```python
from build123d import *

# Parameters (mm, degrees)
SKETCH1_W                                    = 200
SKETCH1_H                                    = 40
BOSS_EXTRUDE1_DEPTH                          = 6
CSK_FOR_M6_COUNTERSUNK_FLAT_HEAD_SCR_2_COUNT = 2
CSK_FOR_M6_COUNTERSUNK_FLAT_HEAD_SCR_2_PITCH = 14
CSK_FOR_M6_COUNTERSUNK_FLAT_HEAD_SCR_3_COUNT = 2
CSK_FOR_M6_COUNTERSUNK_FLAT_HEAD_SCR_3_PITCH = 19.798989873
CSK_FOR_M6_COUNTERSUNK_FLAT_HEAD_SCR_4_COUNT = 2
CSK_FOR_M6_COUNTERSUNK_FLAT_HEAD_SCR_4_PITCH = 14
CHAMFER1_SIZE                                = 2
SKETCH8_R                                    = 5
CUT_EXTRUDE1_DEPTH                           = 103.156742313


with BuildPart() as part:
    # Sketch1 → Boss-Extrude1 (new body)
    with BuildSketch(Plane(origin=(0, 0, 0), x_dir=(1, 0, 0), z_dir=(0, 1, 0))):
        Rectangle(SKETCH1_W, SKETCH1_H)
    extrude(amount=BOSS_EXTRUDE1_DEPTH)

    # Sketch5 → CSK for M6 Countersunk Flat Head Screw1 (revolve, cut)
    with BuildSketch(Plane(origin=(-7, 6, -7), x_dir=(0, 0, 1), z_dir=(1, 0, 0))):
        Polygon((0, 0), (0, 6), (3.3, 6), (3.3, 3.2), (6.5, 0), align=None)
    csk_for_m6_countersunk_flat_head_screw1 = revolve(axis=Axis((-7, 12.35, -7), (0, -1, 0)), mode=Mode.SUBTRACT)

    # CSK for M6 Countersunk Flat Head Scr 2: CSK for M6 Countersunk Flat Head Screw1 ×2
    with Locations(*[(i * CSK_FOR_M6_COUNTERSUNK_FLAT_HEAD_SCR_2_PITCH, 0, 0) for i in range(1, CSK_FOR_M6_COUNTERSUNK_FLAT_HEAD_SCR_2_COUNT)]):
        add(csk_for_m6_countersunk_flat_head_screw1, mode=Mode.SUBTRACT)

    # CSK for M6 Countersunk Flat Head Scr 3: CSK for M6 Countersunk Flat Head Screw1 ×2
    with Locations(*[Vector(0.7071067811865476, 0, 0.7071067811865476) * (i * CSK_FOR_M6_COUNTERSUNK_FLAT_HEAD_SCR_3_PITCH) for i in range(1, CSK_FOR_M6_COUNTERSUNK_FLAT_HEAD_SCR_3_COUNT)]):
        add(csk_for_m6_countersunk_flat_head_screw1, mode=Mode.SUBTRACT)

    # CSK for M6 Countersunk Flat Head Scr 4: CSK for M6 Countersunk Flat Head Screw1 ×2
    with Locations(*[(0, 0, i * CSK_FOR_M6_COUNTERSUNK_FLAT_HEAD_SCR_4_PITCH) for i in range(1, CSK_FOR_M6_COUNTERSUNK_FLAT_HEAD_SCR_4_COUNT)]):
        add(csk_for_m6_countersunk_flat_head_screw1, mode=Mode.SUBTRACT)

    # Chamfer1
    chamfer1_edges = [part.edges().sort_by_distance(p)[0] for p in [
        (-100, 3, 20),
        (-100, 3, -20),
        (100, 3, -20),
        (100, 3, 20),
    ]]
    chamfer(chamfer1_edges, length=CHAMFER1_SIZE)

    # Sketch8 → Cut-Extrude1 (cut, through all)
    with BuildSketch(Plane(origin=(0, 6, 0), x_dir=(1, 0, 0), z_dir=(0, 1, 0))):
        with Locations(Location((-50, 0, 0), (0, 0, 270))):
            Circle(SKETCH8_R)
        with Locations(Location((-80, 0, 0), (0, 0, 270))):
            Circle(SKETCH8_R)
    cut_extrude1 = extrude(amount=-CUT_EXTRUDE1_DEPTH, mode=Mode.SUBTRACT)

    # Mirror1: Cut-Extrude1 across plane
    add(cut_extrude1.mirror(Plane(origin=(0, 0, 0), x_dir=(0, 0, 1), z_dir=(1, 0, 0))), mode=Mode.SUBTRACT)


solid = part.part
```
Source: CAD feature listing. Evaluate the final solid. Frame: model axes, mm. Round coordinates to 2 decimals unless told otherwise and drop trailing zeros. Loops run counter-clockwise (first coordinate to the right, second up) from the corner with the lowest first, then second, coordinate; pieces in that order, holes last.
1. Section query C-C on y = 1.5. Give the number of separate pieces and of enclosed holes in the cut face, and give its area (3 significant figures).
2. Ray query, L1, parallel to Z at x = 7, y = 1.65; L2, parallel to X at y = 4.5, z = 0; L3, parallel to X at y = 1.15, z = 3. Return the intervals inside material, ascending.
3. Section query A-A on z = 7. Output: boundary loops of the cut face in (x, y).
4. Mould query, pull axis X, two halves, no side actions, for faces 1 (the flat face through (100, 3, 0)), 2 (the flat face through (-100, 3, 0)), 3 (the cylindrical face through (-9.23, 1.42, -9.43)). Classes: released by +X, released by -X, zero draft, split by the parting line, or undercut.
5. Section query D-D on x = 50. Output: boundary loops of the cut face in (y, z).
6. Section query B-B on x = -7. Output: boundary loops of the cut face in (y, z), and give its area (3 significant figures).
7. Contact query for flat-ended pins moving along their axis: pin 1 (1.5 mm diameter, centred on x = -33, z = 6.5, fed in from -Y); pin 2 (3 mm diameter, centred on x = 78.5, z = 2, fed in from +Y); pin 3 (7.5 mm diameter, centred on x = -7, z = 7, fed in from +Y). Output: stop coordinate, or through.
Answers below:
1. separate pieces: 1
1. enclosed holes: 8
1. area: 7,540 mm2
2. L1: z = -20 to -10.3, -3.7 to 3.7, 10.3 to 20
2. L2: x = -100 to -85, -75 to -55, -45 to 45, 55 to 75, 85 to 100
2. L3: x = -100 to -84, -76 to -54, -46 to 46, 54 to 76, 84 to 100
3. outline: (-100, 0) - (-10.3, 0) - (-10.3, 2.8) - (-13.5, 6) - (-100, 6) - close; (-3.7, 0) - (3.7, 0) - (3.7, 2.8) - (0.5, 6) - (-0.5, 6) - (-3.7, 2.8) - close; (10.3, 0) - (100, 0) - (100, 6) - (13.5, 6) - (10.3, 2.8) - close
4. face 1: released by +X
4. face 2: released by -X
4. face 3: undercut
5. outline: (0, -20) - (6, -20) - (6, -5) - (0, -5) - close; (0, 5) - (6, 5) - (6, 20) - (0, 20) - close
6. outline: (0, -20) - (6, -20) - (6, -13.5) - (2.8, -10.3) - (0, -10.3) - close; (0, -3.7) - (2.8, -3.7) - (6, -0.5) - (6, 0.5) - (2.8, 3.7) - (0, 3.7) - close; (0, 10.3) - (2.8, 10.3) - (6, 13.5) - (6, 20) - (0, 20) - close
6. area: 140 mm2
7. pin 1: stops at y = 0
7. pin 2: passes through
7. pin 3: stops at y = 3.25
